```python
from build123d import *

# Parameters (mm, degrees)
BOSS_EXTRUDE3_DEPTH = 76.2
CUT_EXTRUDE1_DEPTH  = 63.5
SKETCH6_R           = 7.62
SKETCH6_W           = 10.16
SKETCH6_H           = 10.16
CUT_EXTRUDE2_DEPTH  = 12.7
CUT_EXTRUDE3_REACH  = 263.509
SKETCH12_W          = 15.24
SKETCH12_H          = 7.62


with BuildPart() as part:
    # Sketch1 → Boss-Extrude3 (new body)
    with BuildSketch(Plane(origin=(0, 0, 0), x_dir=(1, 0, 0), z_dir=(0, 1, 0))):
        Polygon((177.8, 76.2), (0, 76.2), (0, 0), (177.8, 0), (177.8, 38.1), (177.8, 63.5), align=None)
        Polygon((0, 152.4), (0, 76.2), (177.8, 76.2), (177.8, 88.9), (177.8, 114.3), (177.8, 152.4), align=None)
        Polygon((228.6, 114.3), (177.8, 152.4), (177.8, 114.3), align=None)
        Polygon((177.8, 114.3), (177.8, 88.9), (190.5, 88.9), (228.6, 88.9), (228.6, 114.3), align=None)
        Polygon((177.8, 38.1), (177.8, 0), (228.6, 38.1), align=None)
        Polygon((190.5, 63.5), (177.8, 63.5), (177.8, 38.1), (228.6, 38.1), (228.6, 63.5), align=None)
        with BuildLine():
            ThreePointArc((190.5, 63.5), (181.519743879, 67.219743879), (177.8, 76.2))
            Line((177.8, 76.2), (177.8, 63.5))
            Line((177.8, 63.5), (190.5, 63.5))
        make_face()
        with BuildLine():
            Line((177.8, 88.9), (177.8, 76.2))
            ThreePointArc((177.8, 76.2), (181.519743879, 85.180256121), (190.5, 88.9))
            Line((190.5, 88.9), (177.8, 88.9))
        make_face()
    extrude(amount=BOSS_EXTRUDE3_DEPTH)

    # Sketch4 → Cut-Extrude1 (cut)
    with BuildSketch(Plane(origin=(0, 76.2, 0), x_dir=(1, 0, 0), z_dir=(0, 1, 0))):
        with BuildLine():
            Line((215.9, 101.6), (215.9, 107.95))
            Line((215.9, 107.95), (173.566666667, 139.7))
            Line((173.566666667, 139.7), (12.7, 139.7))
            Line((12.7, 139.7), (12.7, 12.7))
            Line((12.7, 12.7), (173.566666667, 12.7))
            Line((173.566666667, 12.7), (215.9, 44.45))
            Line((215.9, 44.45), (215.9, 50.8))
            Line((215.9, 50.8), (190.5, 50.8))
            ThreePointArc((190.5, 50.8), (165.1, 76.2), (190.5, 101.6))
            Line((190.5, 101.6), (215.9, 101.6))
        make_face()
    extrude(amount=-CUT_EXTRUDE1_DEPTH, mode=Mode.SUBTRACT)

    # Sketch6 → Cut-Extrude2 (cut)
    with BuildSketch(Plane.ZY):
        with Locations((-78.343351815, 20.32)):
            Circle(SKETCH6_R)
        with Locations((-30.565080817, 20.32)):
            Rectangle(SKETCH6_W, SKETCH6_H)
    extrude(amount=-CUT_EXTRUDE2_DEPTH, mode=Mode.SUBTRACT)

    # Cut-Extrude3: up to this face of the body (flat: up to its plane)
    cut_extrude3_end = Plane(part.part.faces().sort_by_distance((203.2, 44.45, -101.6))[0])
    # Sketch12 → Cut-Extrude3 (cut, up to the picked face)
    with BuildSketch(Plane.XY.offset(-50.8), mode=Mode.PRIVATE) as cut_extrude3_sk1:
        with Locations((201.93, 67.31)):
            Rectangle(SKETCH12_W, SKETCH12_H)
    cut_extrude3_tool1 = split(extrude(cut_extrude3_sk1.sketch, amount=-CUT_EXTRUDE3_REACH, mode=Mode.PRIVATE), bisect_by=cut_extrude3_end, keep=Keep.BOTH, mode=Mode.PRIVATE)
    add(cut_extrude3_tool1.solids().sort_by(Axis((201.93, 67.31, -50.8), (0, 0, -1)))[0], mode=Mode.SUBTRACT)


solid = part.part
```
Read the model definition and answer for the solid it produces. Units are mm, in the model's axes. A direction names the side the tool comes from. Give positions to 0.01 mm unless a question says otherwise; leave off trailing zeros. Loops run counter-clockwise (first coordinate to the right, second up) from the corner with the lowest first, then second, coordinate; pieces in that order, holes last.
Item 1: Find the intervals of material crossed by line 1 along Z through (x, y) = (8.75, 20.32); line 2 along Z through (x, y) = (119, 31.5); line 3 along X through (y, z) = (40, -107.5), in increasing order.
Item 2: The part is cut by section D-D (y = 34.5). Write down the section's boundary in (x, z).
Item 3: The part is cut by section B-B (x = 39.5). Write down the section's boundary in (y, z).
Item 4: Each of these flat-tipped pins is pushed along its axis until it touches: pin 1 Ø3 at (x, z) = (47.5, -132.5) entering from +Y; pin 2 Ø12 at (y, z) = (20.32, -78.34) entering from +X; pin 3 Ø7.5 at (x, y) = (197, 45.5) entering from +Z. Where does it stop, or does it pass through?
Item 5: The part is cut by section C-C (x = 205.5). Write down the section's boundary in (y, z) (3 decimals).
Item 6: The mould has two halves that part along X. Classify faces 1 (the flat face through (6, 20, -35.645)), 2 (the flat face through (0, 38, -77)), 3 (the flat face through (202, 71.12, -57)): released by +X, released by -X, zero draft, split by the parting line, or undercut.
Item 7: For faces 4 (the flat face through (94, 45, -139.7)), 5 (the flat face through (6, 15.24, -31)), 6 (the flat face through (202, 71.12, -95)), determine the directions among +Z, -Z, +X, -X, +Y, -Y from which every point of the face is accessible in a straight line to the end or side of a thin tool.
Item 8: The part is cut by section A-A (y = 20.32). Write down the section's boundary in (x, z).
Taken from the geometry:
1. line 1: z = -152.4 to -85.96, -70.72 to -35.65, -25.49 to 0
1. line 2: z = -152.4 to -139.7, -12.7 to 0
1. line 3: x = 0 to 12.7, 215.9 to 228.6
2. outline: (0, -152.4) - (177.8, -152.4) - (228.6, -114.3) - (228.6, -88.9) - (190.5, -88.9) arc R12.7 cw to (190.5, -63.5) - (228.6, -63.5) - (228.6, -38.1) - (177.8, 0) - (0, 0) - close; hole (12.7, -139.7) - (173.57, -139.7) - (215.9, -107.95) - (215.9, -101.6) - (190.5, -101.6) arc R25.4 cw to (190.5, -50.8) - (215.9, -50.8) - (215.9, -44.45) - (173.57, -12.7) - (12.7, -12.7) - close
3. outline: (0, -152.4) - (76.2, -152.4) - (76.2, -139.7) - (12.7, -139.7) - (12.7, -12.7) - (76.2, -12.7) - (76.2, 0) - (0, 0) - close
4. pin 1: stops at y = 12.7
4. pin 2: stops at x = 180.75
4. pin 3: stops at z = -11.59
5. outline: (0, -131.625) - (76.2, -131.625) - (76.2, -115.75) - (12.7, -115.75) - (12.7, -101.6) - (63.5, -101.6) - (63.5, -88.9) - (0, -88.9) - close; (0, -63.5) - (63.5, -63.5) - (63.5, -50.8) - (12.7, -50.8) - (12.7, -36.65) - (76.2, -36.65) - (76.2, -20.775) - (0, -20.775) - close; (71.12, -101.6) - (76.2, -101.6) - (76.2, -88.9) - (71.12, -88.9) - close; (71.12, -63.5) - (76.2, -63.5) - (76.2, -50.8) - (71.12, -50.8) - close
6. face 1: zero draft
6. face 2: released by -X
6. face 3: undercut
7. face 4: +Y
7. face 5: -X
7. face 6: none
8. outline: (0, -152.4) - (177.8, -152.4) - (228.6, -114.3) - (228.6, -88.9) - (190.5, -88.9) arc R12.7 cw to (190.5, -63.5) - (228.6, -63.5) - (228.6, -38.1) - (177.8, 0) - (0, 0) - (0, -25.49) - (12.7, -25.49) - (12.7, -12.7) - (173.57, -12.7) - (215.9, -44.45) - (215.9, -50.8) - (190.5, -50.8) arc R25.4 ccw to (190.5, -101.6) - (215.9, -101.6) - (215.9, -107.95) - (173.57, -139.7) - (12.7, -139.7) - (12.7, -85.96) - (0, -85.96) - close; (0, -70.72) - (12.7, -70.72) - (12.7, -35.65) - (0, -35.65) - close
